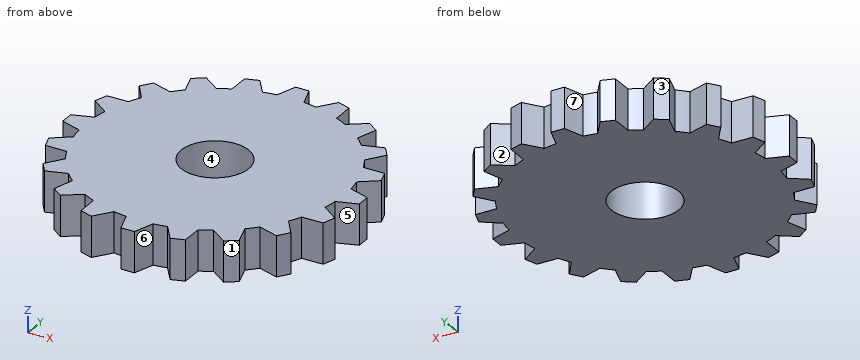
from build123d import *

# Parameters (mm, degrees)
F0_R     = 9.549297
F0_R_2   = 2.5
F2_DEPTH = 3
F3_COUNT = 20
F3_ANGLE = 342


with BuildPart() as f2:
    # F0 (on Top) + F1 (on face) → F2 (new body)
    with BuildSketch(Plane.XY):
        Circle(F0_R)
        Circle(F0_R_2, mode=Mode.SUBTRACT)
    with BuildSketch(Plane.XY):
        with BuildLine():
            ThreePointArc((-1, 9.496792), (0, 9.549297), (1, 9.496792))
            Line((1, 9.496792), (0.5, 10.996792))
            Line((0.5, 10.996792), (-0.5, 10.996792))
            Line((-0.5, 10.996792), (-1, 9.496792))
        make_face()
    extrude(amount=F2_DEPTH)

    # F3: F2 ×20 about axis
    f3_axis = Axis((0, 0, 3), (0, 0, -1))


with BuildPart() as f2_1:
    add(f2.part)
    for i in range(1, F3_COUNT):
        add(f2.part.rotate(f3_axis, i * F3_ANGLE / (F3_COUNT - 1)))


solid = f2_1.part
Check sheet for the modelled part. Datum: model origin and axes. Units: mm. Face numbers are marked on the shaded views. A direction names the side the tool comes from. Round coordinates to 2 decimals unless told otherwise and drop trailing zeros. Write each loop counter-clockwise with the first axis right and the second up, starting at its lowest first coordinate (ties: lowest second). Pieces come first, ordered by that corner, then holes. Notation, with made-up numbers: (10, 33.5) - (62, 33.5) arc R13 cw to (62, 57.5) - close; hole circle Ø8 at (-22.5, -26.5). An arc over 180 degrees is marked (long way). Return JSON: item names as keys, results as strings.
Q1. Access from +Z, -Z, +X, -X, +Y, -Y to the whole of each face (thin tool, end or side, straight path). Record for the marked faces 4, 5, 6 and 7.
Returned:
{"face 4": "+Z, -Z", "face 5": "+Z, -Z, +X", "face 6": "+Z, -Z, -Y", "face 7": "+Z, -Z, +Y"}
Q2. Draft check along X on the marked faces 1, 2 and 3. Enter one of: released by +X, released by -X, zero draft, split by the parting line, or undercut.
Returned:
{"face 1": "released by +X", "face 2": "undercut", "face 3": "released by -X"}
Q3. Depth check by flat-ended pin: P1, Ø1.5, axis at y = 8.5, z = 2.5, coming from the +X side. Enter the tip coordinate at first touch or a pass-through.
Returned:
{"P1": "stops at x = 6.87"}
Q4. Cross-section at C-C (y = 5.75). Record the boundary of the cut face in (x, z), then the cut area to 3 significant figures.
Returned:
{"outline": "(-8.97, 0) - (8.97, 0) - (8.97, 3) - (-8.97, 3) - close", "area": "53.8 mm²"}
Q5. Cross-section at A-A (y = 0). Record the boundary of the cut face in (x, z).
Returned:
{"outline": "(-11, 0) - (-2.5, 0) - (-2.5, 3) - (-11, 3) - close; (2.5, 0) - (11, 0) - (11, 3) - (2.5, 3) - close"}
Q6. Cross-section at D-D (x = -3.5). Record the boundary of the cut face in (y, z), then the cut area to 3 significant figures.
Returned:
{"outline": "(-10.43, 0) - (10.43, 0) - (10.43, 3) - (-10.43, 3) - close", "area": "62.6 mm²"}
Q7. Scan lines: L1, parallel to Y at x = 0, z = 2; L2, parallel to X at y = -9.75, z = 0.15; L3, parallel to X at y = 8.5, z = 2.7. Record each from-to range of solid material in increasing order. Write a range as from..to.
Returned:
{"L1": "y = -11..-2.5, 2.5..11", "L2": "x = -3.88..-2.29, -0.92..0.92, 2.29..3.88", "L3": "x = -6.84..-5.09, -4.35..4.35, 5.09..6.84"}
